Can you work these out from the model? Positions are in its coordinate system, mm. A direction names the side the tool comes from. Round coordinates to 2 decimals unless told otherwise and drop trailing zeros. Write each loop counter-clockwise with the first axis right and the second up, starting at its lowest first coordinate (ties: lowest second). Pieces come first, ordered by that corner, then holes. Notation, with made-up numbers: (-25.75, -17.5) -> (15.25, -17.5) arc R7 cw to (15.25, -7.5) -> close; hole circle Ø8 at (40.25, 73). An arc over 180 degrees is marked (long way). Use CSV: the item, a comma, the result in double quotes.
```python
from build123d import *

# Parameters (mm, degrees)
CROQUIS1_W              = 355.5
CROQUIS1_H              = 463.5
SALIENTE_EXTRUIR1_DEPTH = 200
CROQUIS2_W              = 352
CROQUIS2_H              = 460
CORTAR_EXTRUIR1_DEPTH   = 300
CORTAR_EXTRUIR2_DEPTH   = 470.135707978
CROQUIS4_W              = 463.5
CROQUIS4_H              = 1.75
SALIENTE_EXTRUIR2_DEPTH = 20
CROQUIS5_W              = 463.5
CROQUIS5_H              = 1.75
SALIENTE_EXTRUIR3_DEPTH = 20
CROQUIS6_W              = 355.5
CROQUIS6_H              = 1.75
SALIENTE_EXTRUIR4_DEPTH = 20
CROQUIS7_W              = 355.5
CROQUIS7_H              = 1.75
SALIENTE_EXTRUIR5_DEPTH = 20
CROQUIS8_R              = 2.5
CORTAR_EXTRUIR3_DEPTH   = 20
CROQUIS9_W              = 90
CROQUIS9_H              = 40
CORTAR_EXTRUIR4_DEPTH   = 20
CROQUIS10_W             = 352
CROQUIS10_H             = 1.75
SALIENTE_EXTRUIR6_DEPTH = 98.25


with BuildPart() as part:
    # Croquis1 → Saliente-Extruir1 (new body)
    with BuildSketch(Plane(origin=(0, 0, 0), x_dir=(1, 0, 0), z_dir=(0, 1, 0))):
        Rectangle(CROQUIS1_W, CROQUIS1_H)
    extrude(amount=SALIENTE_EXTRUIR1_DEPTH)

    # Croquis2 → Cortar-Extruir1 (cut)
    with BuildSketch(Plane(origin=(0, 200, 0), x_dir=(1, 0, 0), z_dir=(0, 1, 0))):
        Rectangle(CROQUIS2_W, CROQUIS2_H)
    extrude(amount=-CORTAR_EXTRUIR1_DEPTH, mode=Mode.SUBTRACT)

    # Croquis3 → Cortar-Extruir2 (cut, through all)
    with BuildSketch(Plane.ZY.offset(177.75)):
        Polygon((-131.75, 200), (231.75, 135.905142512), (231.75, 200), align=None)
    extrude(amount=-CORTAR_EXTRUIR2_DEPTH, mode=Mode.SUBTRACT)

    # Croquis4 → Saliente-Extruir2 (add)
    with BuildSketch(Plane.ZY.offset(177.75)):
        with Locations((0, 0.875)):
            Rectangle(CROQUIS4_W, CROQUIS4_H)
    extrude(amount=SALIENTE_EXTRUIR2_DEPTH)

    # Croquis5 → Saliente-Extruir3 (add)
    with BuildSketch(Plane(origin=(177.75, 0, 0), x_dir=(0, 0, -1), z_dir=(1, 0, 0))):
        with Locations((0, 0.875)):
            Rectangle(CROQUIS5_W, CROQUIS5_H)
    extrude(amount=SALIENTE_EXTRUIR3_DEPTH)

    # Croquis6 → Saliente-Extruir4 (add)
    with BuildSketch(Plane(origin=(0, 0, -231.75), x_dir=(-1, 0, 0), z_dir=(0, 0, -1))):
        with Locations((0, 0.875)):
            Rectangle(CROQUIS6_W, CROQUIS6_H)
    extrude(amount=SALIENTE_EXTRUIR4_DEPTH)

    # Croquis7 → Saliente-Extruir5 (add)
    with BuildSketch(Plane.XY.offset(231.75)):
        with Locations((0, 0.875)):
            Rectangle(CROQUIS7_W, CROQUIS7_H)
    extrude(amount=SALIENTE_EXTRUIR5_DEPTH)

    # Croquis8 → Cortar-Extruir3 (cut)
    with BuildSketch(Plane(origin=(0, 1.75, 0), x_dir=(1, 0, 0), z_dir=(0, 1, 0))):
        with Locations(Location((-187.75, 201.75, 0), (0, 0, 270))):
            Circle(CROQUIS8_R)
        with Locations(Location((-187.75, 0, 0), (0, 0, 270))):
            Circle(CROQUIS8_R)
        with Locations(Location((-187.75, 112, 0), (0, 0, 270))):
            Circle(CROQUIS8_R)
        with Locations(Location((187.75, 201.75, 0), (0, 0, 270))):
            Circle(CROQUIS8_R)
        with Locations(Location((187.75, 112, 0), (0, 0, 270))):
            Circle(CROQUIS8_R)
        with Locations(Location((187.75, 0, 0), (0, 0, 270))):
            Circle(CROQUIS8_R)
        with Locations(Location((-187.75, -201.75, 0), (0, 0, 270))):
            Circle(CROQUIS8_R)
        with Locations(Location((-187.75, -112, 0), (0, 0, 270))):
            Circle(CROQUIS8_R)
        with Locations(Location((187.75, -112, 0), (0, 0, 270))):
            Circle(CROQUIS8_R)
        with Locations(Location((187.75, -201.75, 0), (0, 0, 270))):
            Circle(CROQUIS8_R)
        with Locations(Location((0, 241.75, 0), (0, 0, 270))):
            Circle(CROQUIS8_R)
        with Locations(Location((147.75, 241.75, 0), (0, 0, 270))):
            Circle(CROQUIS8_R)
        with Locations(Location((-147.75, 241.75, 0), (0, 0, 270))):
            Circle(CROQUIS8_R)
        with Locations(Location((147.75, -241.75, 0), (0, 0, 270))):
            Circle(CROQUIS8_R)
        with Locations(Location((-147.75, -241.75, 0), (0, 0, 270))):
            Circle(CROQUIS8_R)
    extrude(amount=-CORTAR_EXTRUIR3_DEPTH, mode=Mode.SUBTRACT)

    # Croquis9 → Cortar-Extruir4 (cut)
    with BuildSketch(Plane.XY.offset(231.75)):
        with Locations((118, 48.827571256)):
            Rectangle(CROQUIS9_W, CROQUIS9_H)
        with Locations((0, 48.827571256)):
            Rectangle(CROQUIS9_W, CROQUIS9_H)
        with Locations((-118, 48.827571256)):
            Rectangle(CROQUIS9_W, CROQUIS9_H)
    extrude(amount=-CORTAR_EXTRUIR4_DEPTH, mode=Mode.SUBTRACT)

    # Croquis10 → Saliente-Extruir6 (add)
    with BuildSketch(Plane.XY.offset(-230)):
        with Locations((0, 199.125)):
            Rectangle(CROQUIS10_W, CROQUIS10_H)
    extrude(amount=SALIENTE_EXTRUIR6_DEPTH)


solid = part.part
```
Q1. Suppose I cut it at D-D (x = 117.5). Write out the boundary of the cut face in (y, z).
Resolved:
outline,"(0, -251.75) -> (1.75, -251.75) -> (1.75, -231.75) -> (200, -231.75) -> (200, -131.75) -> (198.25, -131.75) -> (198.25, -230) -> (0, -230) -> close; (0, 230) -> (28.83, 230) -> (28.83, 231.75) -> (1.75, 231.75) -> (1.75, 251.75) -> (0, 251.75) -> close; (68.83, 230) -> (136.21, 230) -> (135.91, 231.75) -> (68.83, 231.75) -> close"
Q2. Suppose I cut it at C-C (z = -166.5). Write out the boundary of the cut face in (x, y).
Resolved:
outline,"(-197.75, 0) -> (-176, 0) -> (-176, 198.25) -> (176, 198.25) -> (176, 0) -> (197.75, 0) -> (197.75, 1.75) -> (177.75, 1.75) -> (177.75, 200) -> (-177.75, 200) -> (-177.75, 1.75) -> (-197.75, 1.75) -> close"
Q3. Suppose I cut it at A-A (x = 170.5). Write out the boundary of the cut face in (y, z).
Resolved:
outline,"(0, -251.75) -> (1.75, -251.75) -> (1.75, -231.75) -> (200, -231.75) -> (200, -131.75) -> (198.25, -131.75) -> (198.25, -230) -> (0, -230) -> close; (0, 230) -> (136.21, 230) -> (135.91, 231.75) -> (1.75, 231.75) -> (1.75, 251.75) -> (0, 251.75) -> close"
Q4. Please list where these lines run through material, in increasing order: probe 1 along Z at (x, y) = (-187.75, 0.5); probe 2 along Z at (x, y) = (187, 1); probe 3 along Z at (x, y) = (147.75, 0.8).
Resolved:
probe 1,"z = -231.75 to -204.25, -199.25 to -114.5, -109.5 to -2.5, 2.5 to 109.5, 114.5 to 199.25, 204.25 to 231.75"
probe 2,"z = -231.75 to -204.13, -199.37 to -114.38, -109.62 to -2.38, 2.38 to 109.62, 114.38 to 199.37, 204.13 to 231.75"
probe 3,"z = -251.75 to -244.25, -239.25 to -230, 230 to 239.25, 244.25 to 251.75"
Q5. Suppose I cut it at B-B (y = 61). Write out the boundary of the cut face in (x, z).
Resolved:
outline,"(-177.75, -231.75) -> (177.75, -231.75) -> (177.75, 231.75) -> (163, 231.75) -> (163, 230) -> (176, 230) -> (176, -230) -> (-176, -230) -> (-176, 230) -> (-163, 230) -> (-163, 231.75) -> (-177.75, 231.75) -> close; (-73, 230) -> (-45, 230) -> (-45, 231.75) -> (-73, 231.75) -> close; (45, 230) -> (73, 230) -> (73, 231.75) -> (45, 231.75) -> close"
Q6. Will these pins go through, and if not, where does the flat tip stop? P1, Ø0.9, axis at x = 8.5, z = 231, coming from the +Y side; P2, Ø8, axis at y = 126.5, z = -181.5, coming from the -X side; P3, Ø0.9, axis at y = 0.5, z = -246.5, coming from the +X side; P4, Ø4, axis at x = 187.75, z = 0, coming from the -Y side.
Resolved:
P1,"stops at y = 136.12"
P2,"stops at x = -177.75"
P3,"stops at x = 177.75"
P4,"passes through"
Q7. If we mould it in two halves opening along X, with no side actions, what happens to faces 4 (the face through (-2, 101, -230)), 5 (the face through (-177.75, 99, 3)), 6 (the face through (177.75, 99, 3)), 7 (the face through (-177, 0, -20))? For each: released by +X, released by -X, zero draft, split by the parting line, or undercut.
Resolved:
face 4,"undercut"
face 5,"released by -X"
face 6,"released by +X"
face 7,"zero draft"
Q8. On a 3-axis mill with a long thin cutter (end or side, diameter ignored), from which of +Z, -Z, +X, -X, +Y, -Y can I reach the whole of each face in a straight line? I mean faces 1 (the face through (-176, 79, 3)), 2 (the face through (188, 1.75, 3)), 3 (the face through (-188, 1.75, -3)). Say none if no direction works.
Resolved:
face 1,"-Y"
face 2,"+Z, -Z, +X, +Y"
face 3,"+Z, -Z, -X, +Y"
